Autodesk Inventor part; units mm, degrees
ref_plane "YZ Plane" through (0, 0, 0) normal (1, 0, 0) x (0, 1, 0)
ref_plane "XZ Plane" through (0, 0, 0) normal (0, 1, 0) x (-1, 0, 0)
ref_plane "XY Plane" through (0, 0, 0) normal (0, 0, 1) x (1, 0, 0)
sketch "Sketch1" plane through (0, 0, 0) normal (0, 0, 1) x (1, 0, 0)
  line L0 (5, 2.8868) -> (5, -2.8868)
  line L1 (5, 2.8868) -> (0, 5.7735)
  line L2 (-5, 2.8868) -> (0, 5.7735)
  line L3 (0, -5.7735) -> (5, -2.8868)
  line L4 (-5, 2.8868) -> (-5, -2.8868)
  line L5 (-5, -2.8868) -> (0, -5.7735)
  point P0 (0, 0)
  point P1 (0, 0)
  point P2 (0, 0)
  point P3 (0, 0)
  point P4 (0, 0)
  point P5 (0, 0)
  dimension "d0" = 120
  dimension "d1" = 120
  dimension "d2" = 120
  dimension "d3" = 120
  dimension "d4" = 120
  dimension "d5" = 120
  dimension "d6" = 10
  dimension "d7" = 5
extrude "Extrusion1" add sketch "Sketch1" along normal blind 5
sketch "Sketch2" plane through (0, 0, 5) normal (0, 0, 1) x (1, 0, 0)
  circle A0 centre (0, 0) radius 2.5
  dimension "d10" = 5
extrude "Extrusion2" add sketch "Sketch2" along normal blind 35
thread "Thread1"
sketch "Sketch3" plane through (0, 0, 40) normal (0, 0, 1) x (1, 0, 0)
  line L0 (0, 0) -> (0, 1.5)
  line L1 (0, 1.5) -> (2, 1.5)
  line L2 (2, 1.5) -> (-2, 1.5)
  circle A0 centre (0, 0) radius 2.5
  circle A1 centre (0, 0) radius 2.5
  dimension "d15" = 1.5
extrude "Extrusion3" cut sketch "Sketch3" against normal blind 19 contours L2 A0 L1 picked at (-1.2006, 1.6398)
properties part number "m5-screw-cut"
Here's how the part is built. I have some questions about the finished solid (model axes, mm). A direction names the side the tool comes from. Round coordinates to 2 decimals unless told otherwise and drop trailing zeros. Order: outer loops, then holes, each group sorted by start corner. A loop starts at its lowest first (then second) coordinate and runs counter-clockwise, first axis right, second up. Notation, with made-up numbers: M -21,64.25 L 17,64.25 A8 ccw 17,79.25 Z; hole C 41,63 d3. An arc over 180 degrees is marked long. One line per question, with ' | ' between items.
1) On a 3-axis mill with a long thin cutter (end or side, diameter ignored), from which of +Z, -Z, +X, -X, +Y, -Y can I reach the whole of each face in a straight line? I mean faces 1 (the flat face through (-5, 0, 2)), 2 (the flat face through (-1.2, -2.5, 5)), 3 (the flat face through (0, 2, 21)). Say none if no direction works.
Checked values:
face 1: +Z, -Z, -X, +Y, -Y | face 2: +Z | face 3: +Z, +X, -X, +Y
2) Imagine slicing it at C-C, the plane x = 0.5. Write out the boundary of the cut face in (y, z).
Checked values:
outline: M -5.48,0 L 5.48,0 L 5.48,5 L 2.45,5 L 2.45,21 L 1.5,21 L 1.5,40 L -2.45,40 L -2.45,5 L -5.48,5 Z
3) I'm going to push flat-ended pins straight in: pin 1 Ø0.5 at (x, y) = (-0.5, 2) entering from +Z; pin 2 Ø3 at (x, y) = (1, 2.5) entering from +Z; pin 3 Ø3 at (x, z) = (1, 13) entering from -Y; pin 4 Ø3 at (y, z) = (2, 14.5) entering from +X. Where does each tip first touch, or does it pass through?
Checked values:
pin 1: stops at z = 21 | pin 2: stops at z = 40 | pin 3: stops at y = -2.5 | pin 4: stops at x = 2.45
4) I need wall thicknesses on line 1 (X direction, y = 1.5, z = 14); line 2 (Z direction, x = -3, y = -2.5); line 3 (Y direction, x = -1.5, z = 3.5). Which ranges of each line are inside material? Lowest first, please.
Checked values:
line 1: x = -2 to 2 | line 2: z = 0 to 5 | line 3: y = -4.91 to 4.91
5) Imagine slicing it at B-B, the plane z = 3. Write out the boundary of the cut face in (x, y), plus the area to 3 significant figures.
Checked values:
outline: M -5,-2.89 L 0,-5.77 L 5,-2.89 L 5,2.89 L 0,5.77 L -5,2.89 Z | area: 86.6 mm²
6) Imagine slicing it at A-A, the plane y = -1.5. Write out the boundary of the cut face in (x, z), plus the area to 3 significant figures.
Checked values:
outline: M -5,0 L 5,0 L 5,5 L 2,5 L 2,40 L -2,40 L -2,5 L -5,5 Z | area: 190 mm²
7) Imagine slicing it at D-D, the plane y = 0. Write out the boundary of the cut face in (x, z), plus the area to 3 significant figures.
Checked values:
outline: M -5,0 L 5,0 L 5,5 L 2.5,5 L 2.5,40 L -2.5,40 L -2.5,5 L -5,5 Z | area: 225 mm²
